Work out the finished part from the listing and answer in its coordinate system (mm). A direction names the side the tool comes from. Coordinates: 2 decimals unless noted, no trailing zeros. Order: outer loops, then holes, each group sorted by start corner. A loop starts at its lowest first (then second) coordinate and runs counter-clockwise, first axis right, second up. Notation, with made-up numbers: (48, -30.75) - (70, -30.75) arc R31 cw to (70, 0.25) - close; hole circle Ø7 at (-9.5, -10). An arc over 180 degrees is marked (long way). Answer as a JSON object with one key per item and string values. Group by question number.
1) The mould has two halves that part along X. Classify faces 1 (the face through (0, -10, 10)), 2 (the face through (-24, -27, 0)), 3 (the face through (-16.283, 7.585, 17.665)): released by +X, released by -X, zero draft, split by the parting line, or undercut.
2) Section C-C (y = 3) is taken. Give the vertices of the cut face in (x, z), plus the area to 3 significant figures.
3) A tool of negligible diameter and unlimited length cuts with its end or side. For faces 4 (the face through (-15.6, -5.9, 14.3)), 5 (the face through (5, 4.343, 0)), 6 (the face through (-20.086, 6.743, -17.694)), from which of +Z, -Z, +X, -X, +Y, -Y can it reach the whole face along a straight path? Write none if from no direction.
4) Section B-B (x = 0) is taken. Give the vertices of the cut face in (y, z), plus the area to 3 significant figures.
5) Each of these flat-tipped pins is pushed along its axis until it touches: P1, Ø10, axis at x = 12, z = 4.5, coming from the +Y side; P2, Ø14, axis at y = -38.5, z = -1.5, coming from the +X side; P3, Ø6, axis at x = 2, z = 7.5, coming from the -Y side. Where does it stop, or does it pass through?
6) Section D-D (x = -11) is taken. Give the vertices of the cut face in (y, z), plus the area to 3 significant figures.
7) Find the intervals of material crossed by line 1 along Y through (x, z) = (-20, 0); line 2 along Z through (x, y) = (0, 1.5); line 3 along Z through (x, y) = (-16, -22.5), in increasing order.
from build123d import *
from OCP.BRepFilletAPI import BRepFilletAPI_MakeChamfer

# Parameters (mm, degrees)
SKETCH1_W                 = 45
SKETCH1_H                 = 19.5
BOSS_EXTRUDE1_DEPTH       = 22.5
M4X0_7_TAPPED_HOLE2_D     = 3.3
BOSS_EXTRUDE3_DEPTH       = 6.3625
M4X0_7_TAPPED_HOLE1_D     = 3.3
M4X0_7_TAPPED_HOLE1_DEPTH = 10
M4X0_7_TAPPED_HOLE1_TIP   = 0.991420021
CUT_EXTRUDE2_DEPTH        = 85
SKETCH2_R                 = 3
CUT_EXTRUDE1_DEPTH        = 50
CUT_EXTRUDE3_DEPTH        = 25
FILLET1_R                 = 1.05
FILLET2_R                 = 1.05
FILLET3_R                 = 0.5
SKETCH12_W                = 25.984765903
SKETCH12_H                = 10.03603234
CUT_EXTRUDE4_DEPTH        = 72.15
CHAMFER1_SIZE             = 14
CHAMFER1_SIZE_2           = 8.082903769


with BuildPart() as part:
    # Sketch1 → Boss-Extrude1 (new, symmetric)
    with BuildSketch(Plane.XY):
        with Locations((0, -0.25)):
            Rectangle(SKETCH1_W, SKETCH1_H)
    extrude(amount=BOSS_EXTRUDE1_DEPTH, both=True)

    # M4x0.7 Tapped Hole2 (through all)
    with Locations(Plane(origin=(0, -10, 0), x_dir=(-1, 0, 0), z_dir=(0, -1, 0))):
        with Locations((0, -17.5), (0, 17.5)):
            Hole(M4X0_7_TAPPED_HOLE2_D / 2)

    # Sketch7 → Boss-Extrude3 (add, symmetric)
    with BuildSketch(Plane.XY):
        Polygon((-22.5, -7.5), (-24, -7.5), (-24, -42.5), (-9, -42.5), (-9, -27.5), (8.5, -10), (-22.5, -10), align=None)
    extrude(amount=BOSS_EXTRUDE3_DEPTH, both=True)

    # M4x0.7 Tapped Hole1
    with Locations(Plane(origin=(-24, 0, 0), x_dir=(0, 0, -1), z_dir=(-1, 0, 0))):
        with Locations((0, 37.5), (0, 22.5)):
            Hole(M4X0_7_TAPPED_HOLE1_D / 2, depth=M4X0_7_TAPPED_HOLE1_DEPTH)
            with Locations((0, 0, -(M4X0_7_TAPPED_HOLE1_DEPTH + M4X0_7_TAPPED_HOLE1_TIP / 2))):  # 118° drill point
                Cone(0, M4X0_7_TAPPED_HOLE1_D / 2, M4X0_7_TAPPED_HOLE1_TIP, mode=Mode.SUBTRACT)

    # Sketch10 → Cut-Extrude2 (cut)
    with BuildSketch(Plane(origin=(0, 0, -6.3625), x_dir=(-1, 0, 0), z_dir=(0, 0, -1))):
        Polygon((22.5, -10), (24, -11.5), (24, -7.5), (22.5, -7.5), align=None)
    extrude(amount=-CUT_EXTRUDE2_DEPTH, mode=Mode.SUBTRACT)

    # Sketch2 → Cut-Extrude1 (cut)
    with BuildSketch(Plane(origin=(0, 9.5, 0), x_dir=(1, 0, 0), z_dir=(0, 1, 0))):
        with Locations(Location((0, 0, 0), (0, 0, 180))):
            Circle(SKETCH2_R)
    extrude(amount=-CUT_EXTRUDE1_DEPTH, mode=Mode.SUBTRACT)

    # Sketch11 → Cut-Extrude3 (cut, symmetric)
    with BuildSketch(Plane.XY):
        Polygon((-17.267020036, 9.5), (-20.520653971, 6.769876965), (-19.170799991, 5.161183635), (-14, 9.5), align=None)
        Polygon((14, 9.5), (17.267020036, 9.5), (20.520653971, 6.769876965), (19.170799991, 5.161183635), align=None)
    extrude(amount=CUT_EXTRUDE3_DEPTH, both=True, mode=Mode.SUBTRACT)

    # Fillet1
    fillet1_edges = [part.edges().sort_by_distance(p)[0] for p in [
        (-19.170799991, 5.161183635, 0),
        (-20.520653971, 6.769876965, 0),
    ]]
    fillet(fillet1_edges, radius=FILLET1_R - 0.0001)  # a hair under: the kernel refuses the full size

    # Fillet2
    fillet2_edges = [part.edges().sort_by_distance(p)[0] for p in [
        (19.170799991, 5.161183635, 0),
        (20.520653971, 6.769876965, 0),
    ]]
    fillet(fillet2_edges, radius=FILLET2_R - 0.0001)  # a hair under: the kernel refuses the full size

    # Fillet3
    fillet3_edges = [part.edges().sort_by_distance(p)[0] for p in [
        (14, 9.5, 0),
        (17.267020036, 9.5, 0),
        (-22.5, 9.5, 0),
        (22.5, 9.5, 0),
        (-17.267020036, 9.5, 0),
        (-14, 9.5, 0),
    ]]
    fillet(fillet3_edges, radius=FILLET3_R)

    # Sketch12 → Cut-Extrude4 (cut)
    with BuildSketch(Plane(origin=(22.5, 0, 0), x_dir=(0, 0, -1), z_dir=(1, 0, 0))):
        with Locations((0.027906174, 9.360607609)):
            Rectangle(SKETCH12_W, SKETCH12_H)
    extrude(amount=-CUT_EXTRUDE4_DEPTH, mode=Mode.SUBTRACT)

    # Chamfer1
    chamfer1_edges_1 = [part.edges().sort_by_distance(p)[0] for p in [
        (-22.5, -10, -14.43125),
    ]]
    chamfer1_side_1 = [part.faces().sort_by_distance(p)[0] for p in [
        (-22.338341925, -10, -14.43125),
    ]]
    chamfer1_edges_2 = [part.edges().sort_by_distance(p)[0] for p in [
        (22.5, -10, 0),
    ]]
    chamfer1_side_2 = [part.faces().sort_by_distance(p)[0] for p in [
        (22.5, -9.838341925, 0),
    ]]
    chamfer1_edges_3 = [part.edges().sort_by_distance(p)[0] for p in [
        (-22.5, -10, 14.43125),
    ]]
    chamfer1_side_3 = [part.faces().sort_by_distance(p)[0] for p in [
        (-22.338341925, -10, 14.43125),
    ]]
    chamfer1 = BRepFilletAPI_MakeChamfer(part.part.solid().wrapped)
    for e in chamfer1_edges_1:
        chamfer1.Add(CHAMFER1_SIZE - 0.0001, CHAMFER1_SIZE_2 - 0.0001, e.wrapped, chamfer1_side_1[0].wrapped)
    for e in chamfer1_edges_2:
        chamfer1.Add(CHAMFER1_SIZE_2 - 0.0001, CHAMFER1_SIZE - 0.0001, e.wrapped, chamfer1_side_2[0].wrapped)
    for e in chamfer1_edges_3:
        chamfer1.Add(CHAMFER1_SIZE - 0.0001, CHAMFER1_SIZE_2 - 0.0001, e.wrapped, chamfer1_side_3[0].wrapped)
    add(Compound.cast(chamfer1.Shape()), mode=Mode.REPLACE)  # a hair under: the kernel refuses the full size


solid = part.part
Report:
{
 "1": {"face 1": "zero draft", "face 2": "released by -X", "face 3": "undercut"},
 "2": {"outline": "(-22.5, -22.5) - (22.5, -22.5) - (22.5, 22.5) - (-22.5, 22.5) - close; hole circle Ø6 at (0, 0); hole circle Ø3.3 at (0, -17.5); hole circle Ø3.3 at (0, 17.5)", "area": "1,980 mm²"},
 "3": {"face 4": "+Z, -X, -Y", "face 5": "+X, -X, +Y", "face 6": "+Z, -Z"},
 "4": {"outline": "(-18.5, -6.36) - (-10, -6.36) - (-10, -15.85) - (9.5, -15.85) - (9.5, -13.02) - (4.34, -13.02) - (4.34, -3) - (-18.5, -3) - close; (-18.5, 3) - (4.34, 3) - (4.34, 12.96) - (9.5, 12.96) - (9.5, 15.85) - (-10, 15.85) - (-10, 6.36) - (-18.5, 6.36) - close; (-10, -22.5) - (9.5, -22.5) - (9.5, -19.15) - (-10, -19.15) - close; (-10, 19.15) - (9.5, 19.15) - (9.5, 22.5) - (-10, 22.5) - close", "area": "586 mm²"},
 "5": {"P1": "stops at y = 4.34", "P2": "stops at x = -9", "P3": "stops at y = -19.28"},
 "6": {"outline": "(-42.5, -6.36) - (-8.56, -6.36) - (-8.56, -22.5) - (9.5, -22.5) - (9.5, -13.02) - (4.34, -13.02) - (4.34, 12.96) - (9.5, 12.96) - (9.5, 22.5) - (-8.56, 22.5) - (-8.56, 6.36) - (-42.5, 6.36) - close", "area": "1,110 mm²"},
 "7": {"line 1": "y = -42.5 to -39.15, -35.85 to -24.15, -20.85 to 4.34", "line 2": "z = -22.5 to -19.15, -15.85 to -3, 3 to 15.85, 19.15 to 22.5", "line 3": "z = -6.36 to -1.65, 1.65 to 6.36"}
}
